Input: part model. Units: mm. Frame: model coordinates. Round coordinates to 2 decimals unless told otherwise and drop trailing zeros. Write each loop counter-clockwise with the first axis right and the second up, starting at its lowest first coordinate (ties: lowest second). Pieces come first, ordered by that corner, then holes. Notation, with made-up numbers: M 48.25,-30.75 L 64.25,-30.75 A11 cw 64.25,-20.75 Z; hole C 68.5,83.5 d9. An arc over 180 degrees is marked long. Answer as CSV lines item,"result". Start each with the question number.
```python
from build123d import *

# Parameters (mm, degrees)
BOSS_EXTRUDE1_DEPTH            = 1.6
BOSS_EXTRUDE2_DEPTH            = 0.1
M2_HOLE1_FIXINGSTRUCTURE_D     = 2.4
M2_HOLE1_FIXINGSTRUCTURE_DEPTH = 200
M2_HOLE1_FIXINGSTRUCTURE_TIP   = 0.721032743


with BuildPart() as part:
    # Sketch1 → Boss-Extrude1 (new body)
    with BuildSketch(Plane.XY):
        with BuildLine():
            Line((-34, 44), (-34, 38))
            ThreePointArc((-34, 38), (-34.146446609, 37.646446609), (-34.5, 37.5))
            Line((-34.5, 37.5), (-40.5, 37.5))
            ThreePointArc((-40.5, 37.5), (-40.853553391, 37.353553391), (-41, 37))
            Line((-41, 37), (-41, -37))
            ThreePointArc((-41, -37), (-40.853553391, -37.353553391), (-40.5, -37.5))
            Line((-40.5, -37.5), (-34.5, -37.5))
            ThreePointArc((-34.5, -37.5), (-34.146446609, -37.646446609), (-34, -38))
            Line((-34, -38), (-34, -44))
            ThreePointArc((-34, -44), (-33.853553391, -44.353553391), (-33.5, -44.5))
            Line((-33.5, -44.5), (33.5, -44.5))
            ThreePointArc((33.5, -44.5), (33.853553391, -44.353553391), (34, -44))
            Line((34, -44), (34, -38))
            ThreePointArc((34, -38), (34.146446609, -37.646446609), (34.5, -37.5))
            Line((34.5, -37.5), (40.5, -37.5))
            ThreePointArc((40.5, -37.5), (40.853553391, -37.353553391), (41, -37))
            Line((41, -37), (41, 37))
            ThreePointArc((41, 37), (40.853553391, 37.353553391), (40.5, 37.5))
            Line((40.5, 37.5), (34.5, 37.5))
            ThreePointArc((34.5, 37.5), (34.146446609, 37.646446609), (34, 38))
            Line((34, 38), (34, 44))
            ThreePointArc((34, 44), (33.853553391, 44.353553391), (33.5, 44.5))
            Line((33.5, 44.5), (-33.5, 44.5))
            ThreePointArc((-33.5, 44.5), (-33.853553391, 44.353553391), (-34, 44))
        make_face()
    extrude(amount=BOSS_EXTRUDE1_DEPTH)

    # Esboço1 → Boss-Extrude2 (add)
    with BuildSketch(Plane.XY.offset(1.6)):
        with BuildLine():
            Line((-29.5, -37.5), (29.5, -37.5))
            ThreePointArc((29.5, -37.5), (33.035533906, -36.035533906), (34.5, -32.5))
            Line((34.5, -32.5), (34.5, 32.5))
            ThreePointArc((34.5, 32.5), (33.035533906, 36.035533906), (29.5, 37.5))
            Line((29.5, 37.5), (-29.5, 37.5))
            ThreePointArc((-29.5, 37.5), (-33.035533906, 36.035533906), (-34.5, 32.5))
            Line((-34.5, 32.5), (-34.5, -32.5))
            ThreePointArc((-34.5, -32.5), (-33.035533906, -36.035533906), (-29.5, -37.5))
        make_face()
    extrude(amount=BOSS_EXTRUDE2_DEPTH)

    # M2 Hole1-FixingStructure
    with Locations(Plane(origin=(0, 0, 0), x_dir=(-1, 0, 0), z_dir=(0, 0, -1))):
        with Locations((-30.5, 40.5), (30.5, 40.5), (-30.5, -40.5), (30.5, -40.5)):
            Hole(M2_HOLE1_FIXINGSTRUCTURE_D / 2, depth=M2_HOLE1_FIXINGSTRUCTURE_DEPTH)
            with Locations((0, 0, -(M2_HOLE1_FIXINGSTRUCTURE_DEPTH + M2_HOLE1_FIXINGSTRUCTURE_TIP / 2))):  # 118° drill point
                Cone(0, M2_HOLE1_FIXINGSTRUCTURE_D / 2, M2_HOLE1_FIXINGSTRUCTURE_TIP, mode=Mode.SUBTRACT)


solid = part.part
```
Item 1: Draft query along X for faces 1 (the face through (31.15, 41.51, 0.81)), 2 (the face through (-37, 0, 1.6)). Return one class per face: +X half, -X half, draft (parallel to the pull), parting line (faces both ways), or undercut.
Item 2: Line query: line 1 (Y direction, x = 30.5, z = 0.7); line 2 (Y direction, x = -37, z = 0.75). Output: solid intervals per line, ascending. Write a range as [from, to].
Item 3: Cut plane B-B, the plane y = 40.5. Return loops of the section in (x, z), plus the area to 3 significant figures.
Item 4: Pin query (flat end, axial travel): pin 1 Ø3 at (x, y) = (-30.5, 40.5) entering from +Z; pin 2 Ø0.8 at (y, z) = (40, 1) entering from -X; pin 3 Ø0.8 at (y, z) = (42, 0.5) entering from +X. Return the tip coordinate at first contact, or that it passes through.
Item 5: Cut plane C-C, the plane x = -30.5. Return loops of the section in (y, z).
Item 6: Cut plane A-A, the plane z = 0.5. Return loops of the section in (x, y), plus the area to 3 significant figures.
Results list:
1,face 1,"undercut"
1,face 2,"draft"
2,line 1,"[-44.5, -41.7], [-39.3, 39.3], [41.7, 44.5]"
2,line 2,"[-37.5, 37.5]"
3,outline,"M -34,0 L -31.7,0 L -31.7,1.6 L -34,1.6 Z; M -29.3,0 L 29.3,0 L 29.3,1.6 L -29.3,1.6 Z; M 31.7,0 L 34,0 L 34,1.6 L 31.7,1.6 Z"
3,area,"101 mm²"
4,pin 1,"z = 1.6"
4,pin 2,"x = -34"
4,pin 3,"x = 34"
5,outline,"M -44.5,0 L -41.7,0 L -41.7,1.6 L -44.5,1.6 Z; M -39.3,0 L 39.3,0 L 39.3,1.6 L 37.4,1.6 L 37.4,1.7 L -37.4,1.7 L -37.4,1.6 L -39.3,1.6 Z; M 41.7,0 L 44.5,0 L 44.5,1.6 L 41.7,1.6 Z"
6,outline,"M -41,-37 A0.5 ccw -40.5,-37.5 L -34.5,-37.5 A0.5 cw -34,-38 L -34,-44 A0.5 ccw -33.5,-44.5 L 33.5,-44.5 A0.5 ccw 34,-44 L 34,-38 A0.5 cw 34.5,-37.5 L 40.5,-37.5 A0.5 ccw 41,-37 L 41,37 A0.5 ccw 40.5,37.5 L 34.5,37.5 A0.5 cw 34,38 L 34,44 A0.5 ccw 33.5,44.5 L -33.5,44.5 A0.5 ccw -34,44 L -34,38 A0.5 cw -34.5,37.5 L -40.5,37.5 A0.5 ccw -41,37 Z; hole C -30.5,-40.5 d2.4; hole C -30.5,40.5 d2.4; hole C 30.5,-40.5 d2.4; hole C 30.5,40.5 d2.4"
6,area,"7,080 mm²"
